Here's how the part is built. I have some questions about the finished solid (model axes, mm). Face numbers are marked on the shaded views. A direction names the side the tool comes from. Round coordinates to 2 decimals unless told otherwise and drop trailing zeros. Write each loop counter-clockwise with the first axis right and the second up, starting at its lowest first coordinate (ties: lowest second). Pieces come first, ordered by that corner, then holes. Notation, with made-up numbers: (14, 10.25) -> (28, 10.25) arc R18 cw to (28, 33.25) -> close; hole circle Ø6 at (-18.5, 61). An arc over 180 degrees is marked (long way). Answer as CSV lines item,"result".
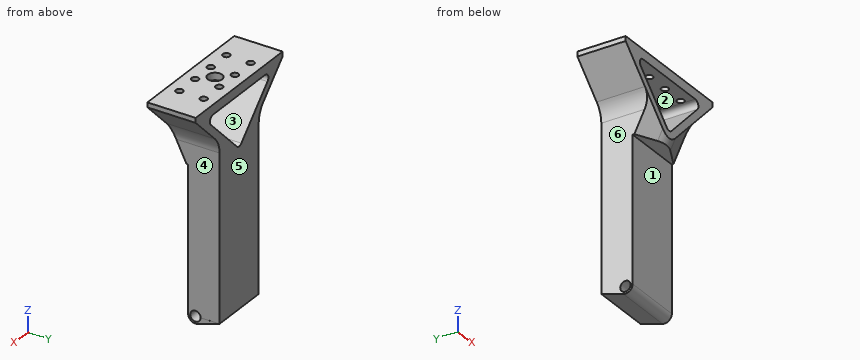
from build123d import *

# Parameters (mm, degrees)
EXTRUDE_1_DEPTH     = 20
SKETCH_2_R          = 1.5
CUT_EXTRUDE_1_DEPTH = 5
SKETCH_3_R          = 3
CUT_EXTRUDE_2_DEPTH = 3
SKETCH_4_W          = 24.99770673
SKETCH_4_H          = 59.73
CUT_EXTRUDE_3_DEPTH = 7
EXTRUDE_2_DEPTH     = 25
SKETCH_6_R          = 2.15
CUT_EXTRUDE_4_DEPTH = 41.24770673
CUT_EXTRUDE_9_DEPTH = 10
FILLET_3_R          = 10
FILLET_4_R          = 10


with BuildPart() as part:
    # 스케치1 → 보스-돌출1 (new body)
    with BuildSketch(Plane(origin=(0, 0, 0), x_dir=(1, 0, 0), z_dir=(0, 1, 0))):
        Polygon((40.24770673, 89.73229327), (15.25229327, 89.73229327), (15.25229327, 17.25229327), (0, 2), (0, 0), (55.5, 0), (55.5, 2), (40.24770673, 17.25229327), align=None)
        with BuildLine():
            Line((11.071067812, 4), (44.428932188, 4))
            ThreePointArc((44.428932188, 4), (46.276691253, 5.234633135), (45.843145751, 7.414213562))
            Line((45.843145751, 7.414213562), (29.164213562, 24.093145751))
            ThreePointArc((29.164213562, 24.093145751), (27.75, 24.678932188), (26.335786438, 24.093145751))
            Line((26.335786438, 24.093145751), (9.656854249, 7.414213562))
            ThreePointArc((9.656854249, 7.414213562), (9.223308747, 5.234633135), (11.071067812, 4))
        make_face(mode=Mode.SUBTRACT)
    extrude(amount=EXTRUDE_1_DEPTH)

    # 스케치2 → 컷-돌출1 (cut)
    with BuildSketch(Plane.XY):
        with Locations((12.75, 15)):
            Circle(SKETCH_2_R)
        with Locations((22.75, 15)):
            Circle(SKETCH_2_R)
        with Locations((32.75, 15)):
            Circle(SKETCH_2_R)
        with Locations((42.75, 15)):
            Circle(SKETCH_2_R)
        with Locations((42.75, 5)):
            Circle(SKETCH_2_R)
        with Locations((32.75, 5)):
            Circle(SKETCH_2_R)
        with Locations((22.75, 5)):
            Circle(SKETCH_2_R)
        with Locations((12.75, 5)):
            Circle(SKETCH_2_R)
    extrude(amount=-CUT_EXTRUDE_1_DEPTH, mode=Mode.SUBTRACT)

    # 스케치3 → 컷-돌출2 (cut)
    with BuildSketch(Plane.XY):
        with Locations((27.75, 10)):
            Circle(SKETCH_3_R)
    extrude(amount=-CUT_EXTRUDE_2_DEPTH, mode=Mode.SUBTRACT)

    # 스케치4 → 컷-돌출3 (cut)
    with BuildSketch(Plane.XZ):
        with Locations((27.748853365, -59.86729327)):
            Rectangle(SKETCH_4_W, SKETCH_4_H)
    extrude(amount=-CUT_EXTRUDE_3_DEPTH, mode=Mode.SUBTRACT)

    # 스케치5 → 보스-돌출2 (add)
    with BuildSketch(Plane.ZY.offset(-15.25229327)):
        with BuildLine():
            Line((-89.73229327, 20), (-92.624677966, 10.804147089))
            ThreePointArc((-92.624677966, 10.804147089), (-92.122576041, 8.184258847), (-89.73229327, 7))
            Line((-89.73229327, 7), (-89.73229327, 20))
        make_face()
    extrude(amount=-EXTRUDE_2_DEPTH)

    # 스케치6 → 컷-돌출4 (cut, through all)
    with BuildSketch(Plane.ZY.offset(-15.25229327)):
        with Locations((-89.734462369, 9.999999216)):
            Circle(SKETCH_6_R)
    extrude(amount=-CUT_EXTRUDE_4_DEPTH, mode=Mode.SUBTRACT)

    # 스케치12 → 컷-돌출9 (cut)
    with BuildSketch(Plane(origin=(9.45846044, -19.103311951, -9.45846044), x_dir=(-0.707106781, 0, -0.707106781), z_dir=(0.405579788, -0.819152044, -0.405579788))):
        Polygon((-16.260212793, 33.305608007), (3.048063237, 33.305608007), (-6.606074778, 45.231574441), align=None)
    cut_extrude_9 = extrude(amount=CUT_EXTRUDE_9_DEPTH, mode=Mode.SUBTRACT)

    # 대칭 복사2: 컷-돌출9 across plane
    add(cut_extrude_9.mirror(Plane(origin=(27.74770673, 0, 0), x_dir=(0, 0, 1), z_dir=(1, 0, 0))), mode=Mode.SUBTRACT)

    # 필렛3
    fillet_3_edges = [part.edges().sort_by_distance(p)[0] for p in [
        (27.74770673, 0.061890187, -29.87729327),
    ]]
    fillet(fillet_3_edges, radius=FILLET_3_R)

    # 필렛4
    fillet_4_edges = [part.edges().sort_by_distance(p)[0] for p in [
        (15.25229327, 10, -17.25229327),
        (40.24770673, 10, -17.25229327),
    ]]
    fillet(fillet_4_edges, radius=FILLET_4_R)


solid = part.part
Item 1: Suppose I cut it at D-D, the plane x = 4. List the corners of the cut face in (y, z) for me.
Results found:
outline,"(0, -6) -> (20, -6) -> (20, 0) -> (0, 0) -> close"
Item 2: I need wall thicknesses on L1, parallel to Y at x = 32.75, z = -1.65; L2, parallel to Y at x = 27.75, z = -1.2; L3, parallel to Z at x = 28, y = 4. Which ranges of each line are inside material? Lowest first, please.
Results found:
L1,"y = 0 to 3.5, 6.5 to 13.5, 16.5 to 20"
L2,"y = 0 to 7, 13 to 20"
L3,"z = -30 to -24.66, -4 to 0"
Item 3: For the marked faces 5 and 6, which set-ups out of +Z, -Z, +X, -X, +Y, -Y let a thin tool reach every point of the face, with its end or its side?
Results found:
face 5,"+Z, -Z, +X, -X, +Y"
face 6,"-Z, -X, +Y, -Y"
Item 4: If we mould it in two halves opening along X, with no side actions, what happens to the marked faces 1, 2, 3 and 4? For each: pulls with the +X half, pulls with the -X half, needs draft (parallel to the pull), parting line crosses it, or undercut.
Results found:
face 1,"needs draft"
face 2,"undercut"
face 3,"undercut"
face 4,"pulls with the +X half"
Item 5: Suppose I cut it at B-B, the plane y = 15. State how many separate pieces and enclosed holes the cut face has, then the cut area to 3 significant figures.
Results found:
separate pieces,"4"
enclosed holes,"0"
area,"2,080 mm²"
Item 6: Suppose I cut it at C-C, the plane z = -10. List the corners of the cut face in (x, y) for me.
Results found:
outline,"(8, 0) -> (12.24, 0) -> (12.24, 20) -> (8, 20) -> close; (43.26, 0) -> (47.5, 0) -> (47.5, 20) -> (43.26, 20) -> close"
Item 7: Will these pins go through, and if not, where does the flat tip stop? pin 1 (1.5 mm diameter, centred on y = 11.5, z = -52, fed in from -X); pin 2 (3.5 mm diameter, centred on x = 42.75, y = 5, fed in from +Z); pin 3 (5 mm diameter, centred on x = 32.75, y = 5, fed in from -Z); pin 4 (3 mm diameter, centred on x = 24.5, y = 2.5, fed in from -Z).
Results found:
pin 1,"stops at x = 15.25"
pin 2,"stops at z = 0"
pin 3,"stops at z = -91.39"
pin 4,"stops at z = -30"
Item 8: Suppose I cut it at A-A, the plane x = 27.75. List the corners of the cut face in (y, z) for me.
Results found:
outline,"(0, -27.63) -> (1.17, -30) -> (7, -30) -> (7, -89.73) arc R3 ccw to (10.8, -92.62) -> (20, -89.73) -> (20, -24.68) -> (0, -24.68) -> close; (0, -4) -> (20, -4) -> (20, 0) -> (13, 0) -> (13, -3) -> (7, -3) -> (7, 0) -> (0, 0) -> close; hole circle Ø4.3 at (10, -89.73)"
